Autodesk Inventor part; units mm, degrees
ref_plane "YZ Plane" through (0, 0, 0) normal (1, 0, 0) x (0, 1, 0)
ref_plane "XZ Plane" through (0, 0, 0) normal (0, 1, 0) x (-1, 0, 0)
ref_plane "XY Plane" through (0, 0, 0) normal (0, 0, 1) x (1, 0, 0)
sketch "スケッチ2" plane through (0, 0, 0) normal (1, 0, 0) x (0, 1, 0)
  line L0 (-50, 41.625) -> (0, 41.625)
  line L1 (0, 41.625) -> (0, 31.625)
  line L2 (0, 31.625) -> (-50, 31.625)
  line L3 (-50, 31.625) -> (-50, 41.625)
  line L4 (0, 31.625) -> (-8, 31.625)
  line L5 (-8, 31.625) -> (-8, 0)
  line L6 (-8, 0) -> (0, 0)
  line L7 (0, 0) -> (0, 31.625)
  circle A0 centre (-20, 36.625) radius 2.25
  circle A1 centre (-35, 36.625) radius 2.25
  line L8 (-8, 31.625) -> (0, 31.625)
  line L9 (0, 31.625) -> (0, 54)
  line L10 (0, 54) -> (-8, 54)
  line L11 (-8, 54) -> (-8, 31.625)
  point P0 (-8, 31.625)
  point P1 (-8, 41.625)
  point P2 (0, 41.625)
  dimension "d7" = 50
  dimension "d8" = 10
  dimension "d10" = 8
  dimension "d11" = 4.5
  dimension "d12" = 4.5
  dimension "d13" = 15
  dimension "d14" = 20
  dimension "d15" = 5
  dimension "d16" = 5
  dimension "d27" = 54
  dimension "d28" = 12.375
extrude "押し出し2" add sketch "スケッチ2" along normal blind 6 contours L0 L11 L2 L3
extrude "押し出し5" add sketch "スケッチ2" along normal blind 70 contours L11 L10 L9 L0 | L0 L1 L2 L11 | L2 L7 L6 L5
sketch "スケッチ4" plane through (0, 0, 54) normal (0, 1, 0) x (1, 0, 0)
  line L0 (70, 54) -> (70, 0)
  line L1 (70, 15) -> (15, 0)
  line L2 (15, 0) -> (15, 54)
  line L3 (15, 54) -> (70, 39)
  line L4 (0, 54) -> (70, 54)
  line L5 (0, 0) -> (70, 0)
  line L6 (0, 54) -> (0, 0)
  line L7 (0, 22.375) -> (0, 54)
  line L8 (0, 54) -> (8.9192, 54)
  line L9 (8.9192, 54) -> (8.9192, 31.7036)
  line L10 (8.9192, 31.7036) -> (0, 31.7036)
  line L11 (0, 31.7036) -> (0, 54)
  dimension "d31" = 15
  dimension "d32" = 15
  dimension "d33" = 15
extrude "押し出し6" cut sketch "スケッチ4" against normal blind 8 contours L0 L3 L4 | L0 L5 L1 | L9 L10 L6 L4
sketch "スケッチ5" plane through (0, -8, 41.625) normal (0, -1, 0) x (1, 0, 0)
  line L0 (70, -2.625) -> (70, -26.625)
  line L1 (15, -41.625) -> (70, -26.625)
  line L2 (70, -2.625) -> (15, 12.375)
  line L3 (70, -26.625) -> (15, -41.625)
  line L4 (70.01, -26.6223) -> (70.01, -2.6277)
  line L5 (70.01, -26.6223) -> (70, -26.625)
  line L6 (70.01, -2.6277) -> (70, -2.625)
  point P0 (0, -41.625)
  dimension "d36" = 0.01
extrude "押し出し7" add sketch "スケッチ5" against normal blind 8
equation "\"d32\" = d31"
equation "\"d33\" = d31"
properties part number "right-nail" material "ABS プラスチック"
Geometry check sheet. Reference: the model listing, model coordinates, mm. A direction names the side the tool comes from. Give positions to 0.01 mm unless a question says otherwise; leave off trailing zeros. Order: outer loops, then holes, each group sorted by start corner. A loop starts at its lowest first (then second) coordinate and runs counter-clockwise, first axis right, second up. Notation, with made-up numbers: (61, -19.75) - (91, -19.75) arc R17 cw to (91, -0.75) - close; hole circle Ø7 at (69, 52.25). An arc over 180 degrees is marked (long way). Write item = value, one per line. Start each with the question number.
1) Draft check along Y on faces 6 (the flat face through (42.885, -3.944, 46.395)), 7 (the flat face through (3, -50, 37)), 8 (the cylindrical face through (2.96, -33.79, 34.73)). Enter one of: released by +Y, released by -Y, zero draft, split by the parting line, or undercut.
2) Section check A-A (y = -20). Enter the section's corners in (x, z) (3 decimals), then the cut area to 3 significant figures.
3) Gauge pin test, flat ends, axial feed: pin 1 Ø3 at (x, y) = (2.5, -38.5) entering from +Z (3 decimals); pin 2 Ø3 at (y, z) = (-26, 38) entering from +X; pin 3 Ø6.5 at (y, z) = (-6, 13) entering from -X. Record the tip position at first contact, or that the pin passes through.
4) Access from +Z, -Z, +X, -X, +Y, -Y to the whole of each face (thin tool, end or side, straight path). Record for faces 1 (the flat face through (0, -18, 38)), 2 (the flat face through (8.919, -4, 11)), 3 (the flat face through (3, -29, 41.625)), 4 (the flat face through (3, -29, 31.625)), 5 (the flat face through (6, -29, 37)).
5) Section check C-C (z = 16.5). Enter the section's corners in (x, y), then the cut area to 3 significant figures.
6) Scan lines: L1, parallel to Z at x = 2, y = -20 (3 decimals); L2, parallel to Y at x = 27, z = 47; L3, parallel to Z at x = 6.5, y = -5.5. Record each from-to range of solid material in increasing order.
7) Section check D-D (x = 53). Enter the section's corners in (y, z).
Geometry check:
q1.face_6 = zero draft
q1.face_7 = released by -Y
q1.face_8 = undercut
q2.outline = (0, 31.625) - (6, 31.625) - (6, 34.375) - (0, 34.375) - close; (0, 38.875) - (6, 38.875) - (6, 41.625) - (0, 41.625) - close
q2.area = 33.0 mm2
q3.pin_1 = 41.625
q3.pin_2 = 6
q3.pin_3 = 8.92
q4.face_1 = +Z, -Z, -X, +Y, -Y
q4.face_2 = -Z, -X, +Y, -Y
q4.face_3 = +Z, +X, -X, -Y
q4.face_4 = -Z, +X, -X, -Y
q4.face_5 = +Z, -Z, +X, -Y
q5.outline = (8.92, -8) - (70.01, -8) - (70.01, 0) - (8.92, 0) - close
q5.area = 489 mm2
q6.L1 = 31.625 to 34.375, 38.875 to 41.625
q6.L2 = -8 to 0
q6.L3 = 22.3 to 54
q7.outline = (-8, 10.36) - (0, 10.36) - (0, 43.64) - (-8, 43.64) - close
